Part model, mm, in its own coordinate system. A direction names the side the tool comes from. Round coordinates to 2 decimals unless told otherwise and drop trailing zeros. Order: outer loops, then holes, each group sorted by start corner. A loop starts at its lowest first (then second) coordinate and runs counter-clockwise, first axis right, second up. Notation, with made-up numbers: (23, 75.5) -> (59, 75.5) arc R23 cw to (59, 84.5) -> close; hole circle Ø6 at (67.25, -33.75). An arc over 180 degrees is marked (long way). Return JSON: item names as keys, results as strings. Group by question number.
from build123d import *

# Parameters (mm, degrees)
BOSS_EXTRUDE1_DEPTH = 6.71
SKETCH2_W           = 1.5
SKETCH2_H           = 5.51
CUT_EXTRUDE1_DEPTH  = 51
SKETCH3_R           = 7.9502
CUT_EXTRUDE2_DEPTH  = 3.81
SKETCH4_W           = 136.2
SKETCH4_H           = 1.4
CUT_EXTRUDE3_DEPTH  = 7.71
SKETCH5_R           = 2.65
CUT_EXTRUDE4_DEPTH  = 3.9
FILLET1_R           = 0.3


with BuildPart() as part:
    # Sketch1 → Boss-Extrude1 (new body)
    with BuildSketch(Plane.XY):
        with BuildLine():
            Line((-63.1, 2.5), (-12.247448714, 2.5))
            ThreePointArc((-12.247448714, 2.5), (0, 12.5), (12.247448714, 2.5))
            Line((12.247448714, 2.5), (63.1, 2.5))
            Line((63.1, 2.5), (63.1, 25))
            Line((63.1, 25), (68.1, 25))
            Line((68.1, 25), (68.1, -25))
            Line((68.1, -25), (63.1, -25))
            Line((63.1, -25), (63.1, -2.5))
            Line((63.1, -2.5), (12.247448714, -2.5))
            ThreePointArc((12.247448714, -2.5), (0, -12.5), (-12.247448714, -2.5))
            Line((-12.247448714, -2.5), (-63.1, -2.5))
            Line((-63.1, -2.5), (-63.1, -25))
            Line((-63.1, -25), (-68.1, -25))
            Line((-68.1, -25), (-68.1, 25))
            Line((-68.1, 25), (-63.1, 25))
            Line((-63.1, 25), (-63.1, 2.5))
        make_face()
    extrude(amount=BOSS_EXTRUDE1_DEPTH)

    # Sketch2 → Cut-Extrude1 (cut, through all)
    with BuildSketch(Plane.XZ.offset(25)):
        with Locations((67.35, 3.955)):
            Rectangle(SKETCH2_W, SKETCH2_H)
        with Locations((-67.35, 3.955)):
            Rectangle(SKETCH2_W, SKETCH2_H)
    extrude(amount=-CUT_EXTRUDE1_DEPTH, mode=Mode.SUBTRACT)

    # Sketch3 → Cut-Extrude2 (cut)
    with BuildSketch(Plane.XY.offset(6.71)):
        Circle(SKETCH3_R)
    extrude(amount=-CUT_EXTRUDE2_DEPTH, mode=Mode.SUBTRACT)

    # Sketch4 → Cut-Extrude3 (cut, through all)
    with BuildSketch(Plane.XY.offset(6.71)):
        with Locations((0, 24.3)):
            Rectangle(SKETCH4_W, SKETCH4_H)
    extrude(amount=-CUT_EXTRUDE3_DEPTH, mode=Mode.SUBTRACT)

    # Sketch5 → Cut-Extrude4 (cut, through all)
    with BuildSketch(Plane.XY.offset(2.9)):
        Circle(SKETCH5_R)
    extrude(amount=-CUT_EXTRUDE4_DEPTH, mode=Mode.SUBTRACT)

    # Fillet1
    fillet1_edges = [part.edges().sort_by_distance(p)[0] for p in [
        (-68.1, -0.7, 1.2),
        (-68.1, -0.7, 0),
    ]]
    fillet(fillet1_edges, radius=FILLET1_R)


solid = part.part
(1) Saw through at C-C, the plane x = 0. List the corners of the cut face in (y, z).
(2) Tool access for faces 1 (the cylindrical face through (-1.72, -7.76, 4.83)), 2 (the flat face through (63.1, 13, 3)), 3 (the flat face through (66.6, -1, 4)), 4 (the flat face through (63.1, -14, 3)): list every direction of +Z, -Z, +X, -X, +Y, -Y with a clear straight run to the whole face (end or side of a thin tool).
(3) Saw through at A-A, the plane y = 0. List the corners of the cut face in (x, z), and give its area (3 significant figures).
(4) Mould opens along X. For faces 5 (the flat face through (-66.6, -1, 4)), 6 (the flat face through (-63.1, -14, 3)), 7 (the flat face through (0, 3, 0)) say: pulls with the +X half, pulls with the -X half, needs draft (parallel to the pull), parting line crosses it, or undercut.
(5) Pin check, flat tips, straight feed: P1, Ø3, axis at y = 4, z = 3, coming from the +X side; P2, Ø1, axis at x = -28.5, z = 2, coming from the +Y side; P3, Ø3.5, axis at x = -29, z = 2, coming from the -Y side; P4, Ø3, axis at x = 0, y = 0, coming from the -Z side. Stop position of each tip, or through.
(6) Saw through at B-B, the plane z = 4.75. List the corners of the cut face in (x, y).
(7) Saw through at D-D, the plane y = 6.5. List the corners of the cut face in (x, z), and give its area (3 significant figures).
(8) Probe L1, parallel to X at y = -3.5, z = 4; L2, parallel to X at y = 16, z = 5.5; L3, parallel to X at y = -22, z = 0.5. List the from-to ranges inside material, lowest first. Write a range as [from, to].
Results are:
{
 "1": {"outline": "(-12.5, 0) -> (-2.65, 0) -> (-2.65, 2.9) -> (-7.95, 2.9) -> (-7.95, 6.71) -> (-12.5, 6.71) -> close; (2.65, 0) -> (12.5, 0) -> (12.5, 6.71) -> (7.95, 6.71) -> (7.95, 2.9) -> (2.65, 2.9) -> close"},
 "2": {"face 1": "+Z", "face 2": "+Z, -Z, +Y", "face 3": "+Z, +X, +Y, -Y", "face 4": "+Z, -Z, -Y"},
 "3": {"outline": "(-68.1, 0.3) arc R0.3 ccw to (-67.8, 0) -> (-2.65, 0) -> (-2.65, 2.9) -> (-7.95, 2.9) -> (-7.95, 6.71) -> (-66.6, 6.71) -> (-66.6, 1.2) -> (-67.8, 1.2) arc R0.3 ccw to (-68.1, 0.9) -> close; (2.65, 0) -> (68.1, 0) -> (68.1, 1.2) -> (66.6, 1.2) -> (66.6, 6.71) -> (7.95, 6.71) -> (7.95, 2.9) -> (2.65, 2.9) -> close", "area": "821 mm^2"},
 "4": {"face 5": "pulls with the -X half", "face 6": "undercut", "face 7": "needs draft"},
 "5": {"P1": "stops at x = 66.6", "P2": "stops at y = 2.5", "P3": "stops at y = -2.5", "P4": "passes through"},
 "6": {"outline": "(-66.6, -25) -> (-63.1, -25) -> (-63.1, -2.5) -> (-12.25, -2.5) arc R12.5 ccw to (12.25, -2.5) -> (63.1, -2.5) -> (63.1, -25) -> (66.6, -25) -> (66.6, 23.6) -> (63.1, 23.6) -> (63.1, 2.5) -> (12.25, 2.5) arc R12.5 ccw to (-12.25, 2.5) -> (-63.1, 2.5) -> (-63.1, 23.6) -> (-66.6, 23.6) -> close; hole circle Ø15.9 at (0, 0)"},
 "7": {"outline": "(-68.1, 0.3) arc R0.3 ccw to (-67.8, 0) -> (-63.1, 0) -> (-63.1, 6.71) -> (-66.6, 6.71) -> (-66.6, 1.2) -> (-67.8, 1.2) arc R0.3 ccw to (-68.1, 0.9) -> close; (-10.68, 0) -> (10.68, 0) -> (10.68, 6.71) -> (4.58, 6.71) -> (4.58, 2.9) -> (-4.58, 2.9) -> (-4.58, 6.71) -> (-10.68, 6.71) -> close; (63.1, 0) -> (68.1, 0) -> (68.1, 1.2) -> (66.6, 1.2) -> (66.6, 6.71) -> (63.1, 6.71) -> close", "area": "159 mm^2"},
 "8": {"L1": "x = [-66.6, -63.1], [-12, -7.14], [7.14, 12], [63.1, 66.6]", "L2": "x = [-66.6, -63.1], [63.1, 66.6]", "L3": "x = [-68.1, -63.1], [63.1, 68.1]"}
}
